Geometry check sheet. Reference: the model listing, model coordinates, mm. Face numbers are marked on the shaded views. A direction names the side the tool comes from. Coordinates: 2 decimals unless noted, no trailing zeros. Order: outer loops, then holes, each group sorted by start corner. A loop starts at its lowest first (then second) coordinate and runs counter-clockwise, first axis right, second up. Notation, with made-up numbers: M -23.5,-18.5 L 6.5,-18.5 A21 ccw 6.5,0.5 Z; hole C 1,55 d11. An arc over 180 degrees is marked long. One line per item, written item: value. Start each with the question number.
1) Sectioned sample at C-C, the plane x = 17.5. Enter the section's corners in (y, z).
2) Thickness scan on L1, parallel to Z at x = 30, y = 32.7; L2, parallel to Z at x = 30, y = 20; L3, parallel to Y at x = 12, z = 4.25. Record the ranges inside material, lowest first. Write a range as from..to.
3) Access from +Z, -Z, +X, -X, +Y, -Y to the whole of each face (thin tool, end or side, straight path). Record for the marked faces 4 and 5.
4) Draft check along X on the marked faces 1, 2 and 3. Enter one of: pulls with the +X half, pulls with the -X half, needs draft (parallel to the pull), parting line crosses it, or undercut.
5) Sectioned sample at B-B, the plane y = 7.4. Enter the section's corners in (x, z), then the cut area to 3 significant figures.
6) Sectioned sample at A-A, the plane z = 11. State how many separate pieces and enclosed holes the cut face has, then the cut area to 3 significant figures.
7) Sectioned sample at D-D, the plane z = 4.5. Enter the section's corners in (x, y), then the cut area to 3 significant figures.
8) Go/stop test with flat-tipped pins: P1, Ø6, axis at x = 30, z = 11, coming from the +Y side; P2, Ø3, axis at x = 32, z = 19, coming from the -Y side; P3, Ø12, axis at y = 6, z = 9.5, coming from the +X side. Record where each tip stops, or that it passes through.
```python
from build123d import *

# Parameters (mm, degrees)
PAD_DEPTH       = 22
SKETCH001_R     = 3.4
POCKET_DEPTH    = 15.001
SKETCH002_W     = 4.8
SKETCH002_H     = 11.4
POCKET001_DEPTH = 13.5
SKETCH003_R     = 2.4
POCKET002_DEPTH = 35.801
SKETCH004_R     = 3.9
POCKET003_DEPTH = 4
POCKET004_DEPTH = 4.2
FILLET_R        = 19
FILLET001_R     = 3
FILLET002_R     = 5


with BuildPart() as part:
    # Sketch → Pad (new body)
    with BuildSketch(Plane.XY):
        Polygon((0, 0), (0, 14.8), (38, 14.8), (38, 35.8), (-15, 35.8), (-15, 0), align=None)
    extrude(amount=PAD_DEPTH)

    # Sketch001 (on Face1 of Pad) → Pocket (cut, through all)
    with BuildSketch(Plane.YZ):
        with Locations((7.4, 11)):
            Circle(SKETCH001_R)
    extrude(amount=-POCKET_DEPTH, mode=Mode.SUBTRACT)

    # Sketch002 (on Face8 of Pocket) → Pocket001 (cut)
    with BuildSketch(Plane.YZ.offset(38)):
        with Locations((25.3, 11)):
            Rectangle(SKETCH002_W, SKETCH002_H)
    extrude(amount=-POCKET001_DEPTH, mode=Mode.SUBTRACT)

    # Sketch003 (on Face9 of Pocket001) → Pocket002 (cut, through all)
    with BuildSketch(Plane(origin=(0, 35.8, 0), x_dir=(-1, 0, 0), z_dir=(0, 1, 0))):
        with Locations((-30, 11)):
            Circle(SKETCH003_R)
    extrude(amount=-POCKET002_DEPTH, mode=Mode.SUBTRACT)

    # Sketch004 (on Face9 of Pocket002) → Pocket003 (cut)
    with BuildSketch(Plane(origin=(0, 35.8, 0), x_dir=(-1, 0, 0), z_dir=(0, 1, 0))):
        with Locations((-30, 11)):
            Circle(SKETCH004_R)
    extrude(amount=-POCKET003_DEPTH, mode=Mode.SUBTRACT)

    # Sketch005 (on Face5 of Pocket003) → Pocket004 (cut)
    with BuildSketch(Plane.XZ.offset(-14.8)):
        Polygon((30, 6.785343), (33.65, 8.892672), (33.65, 13.107328), (30, 15.214657), (26.35, 13.107328), (26.35, 8.892672), align=None)
    extrude(amount=-POCKET004_DEPTH, mode=Mode.SUBTRACT)

    # Fillet
    fillet_edges = [part.edges().sort_by_distance(p)[0] for p in [
        (-15, 35.8, 11),
    ]]
    fillet(fillet_edges, radius=FILLET_R)

    # Fillet001
    fillet001_edges = [part.edges().sort_by_distance(p)[0] for p in [
        (-15, 8.4, 22),
        (-15, 8.4, 0),
    ]]
    fillet(fillet001_edges, radius=FILLET001_R)

    # Fillet002
    fillet002_edges = [part.edges().sort_by_distance(p)[0] for p in [
        (24.5, 25.3, 16.7),
        (24.5, 25.3, 5.3),
    ]]
    fillet(fillet002_edges, radius=FILLET002_R)


solid = part.part
```
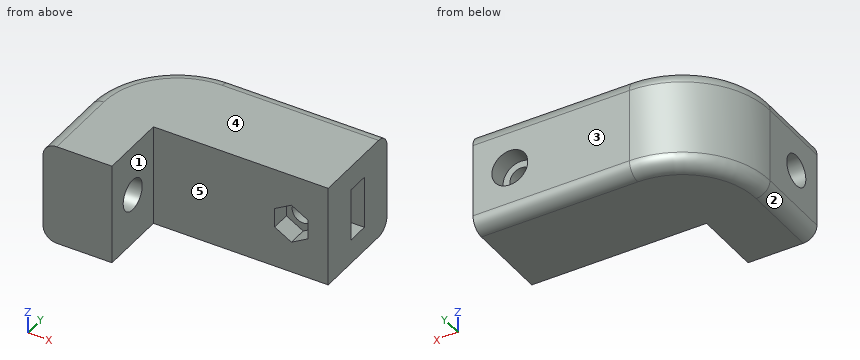
Final values:
1. outline: M 14.8,0 L 32.8,0 A3 ccw 35.8,3 L 35.8,19 A3 ccw 32.8,22 L 14.8,22 Z
2. L1: z = 0..7.1, 14.9..22
2. L2: z = 0..8.6, 13.4..22
2. L3: y = 14.8..35.8
3. face 4: +Z, +X, -X, +Y, -Y
3. face 5: +Z, -Z, +X, -Y
4. face 1: pulls with the +X half
4. face 2: pulls with the -X half
4. face 3: needs draft
5. outline: M -15,3 A3 ccw -12,0 L 0,0 L 0,7.6 L -15,7.6 Z; M -15,14.4 L 0,14.4 L 0,22 L -12,22 A3 ccw -15,19 Z
5. area: 224 mm^2
6. separate pieces: 4
6. enclosed holes: 0
6. area: 990 mm^2
7. outline: M -15,0 L 0,0 L 0,14.8 L 38,14.8 L 38,35.8 L 4,35.8 A19 ccw -15,16.8 Z
7. area: 1,260 mm^2
8. P1: stops at y = 31.8
8. P2: stops at y = 14.8
8. P3: stops at x = 0
